Geometry: see drawing. Coordinates: mm, zero at the bounding-box minimum. A direction names the side the tool comes from. Coordinates: 2 decimals unless noted, no trailing zeros. Order: outer loops, then holes, each group sorted by start corner. A loop starts at its lowest first (then second) coordinate and runs counter-clockwise, first axis right, second up.
Item 1: Section D-D on y = 6. Return the cut outline in (x, z), then the cut area to 3 significant figures.
Item 2: Section A-A on x = 11.25. Return the cut outline in (y, z), then the cut area to 3 significant figures.
Item 3: Mould query, pull axis X, two halves, no side actions, for the marked faces 1, 2 and 3. Classes: released by +X, released by -X, zero draft, split by the parting line, or undercut.
Item 4: Reachability of the marked faces 4, 5, 6, 7 and 8 from +Z, -Z, +X, -X, +Y, -Y: full face, straight path, thin tool, end or side. Return the list, or none.
Item 5: Contact query for flat-ended pins moving along their axis: P1, Ø2, axis at y = 11, z = 9.5, coming from the -X side (3 decimals); P2, Ø1.2, axis at y = 9, z = 11, coming from the +X side (3 decimals); P3, Ø1.2, axis at x = 10.5, y = 9, coming from the +Z side; P4, Ø4, axis at x = 12, z = 2.5, coming from the -Y side. Output: stop coordinate, or through.
Item 6: Section C-C on z = 11. Return the cut outline in (x, y) (3 decimals), then the cut area to 3 significant figures.
Item 7: Section B-B on y = 10. Return the cut outline in (x, z) (3 decimals), then the cut area to 3 significant figures.
Item 8: Ray query, line 1 (Z direction, x = 6, y = 9.25); line 2 (X direction, y = 11, z = 10.75) (3 decimals); line 3 (Z direction, x = 12, y = 2). Return the intervals inside material, ascending.
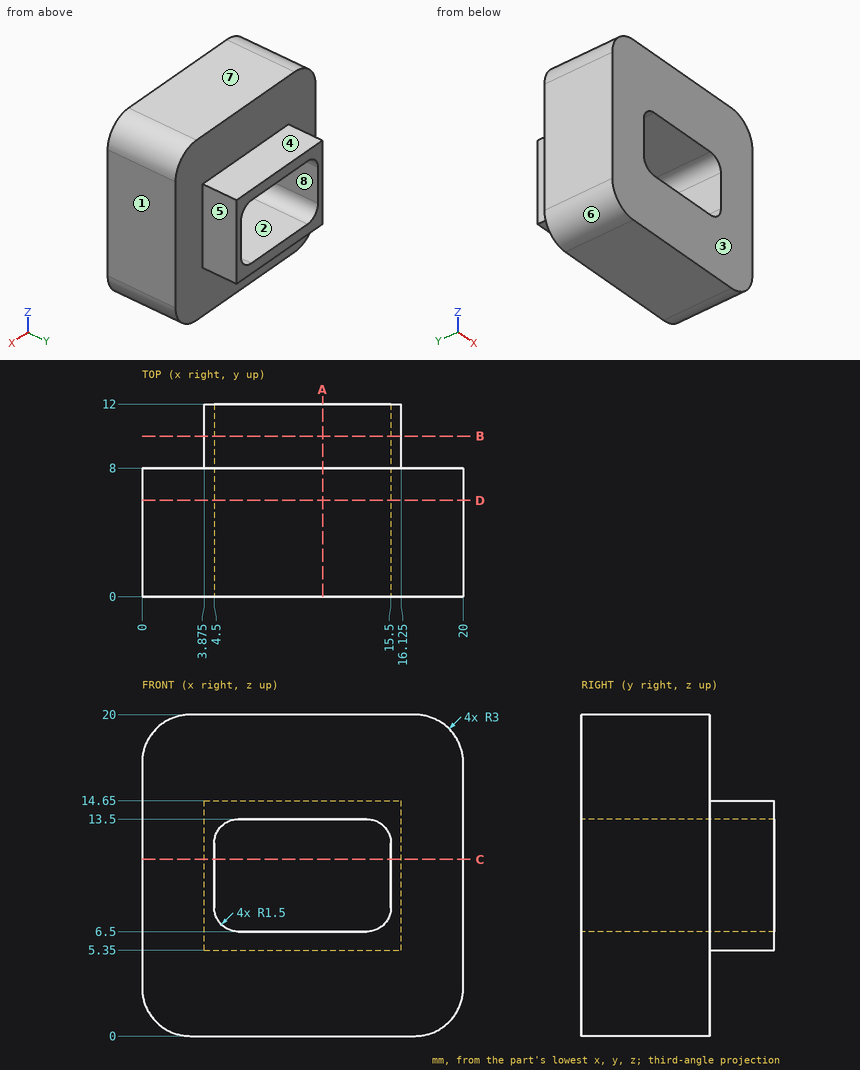
Answer list:
1. outline: (0, 3) arc R3 ccw to (3, 0) - (17, 0) arc R3 ccw to (20, 3) - (20, 17) arc R3 ccw to (17, 20) - (3, 20) arc R3 ccw to (0, 17) - close; hole (4.5, 8) arc R1.5 ccw to (6, 6.5) - (14, 6.5) arc R1.5 ccw to (15.5, 8) - (15.5, 12) arc R1.5 ccw to (14, 13.5) - (6, 13.5) arc R1.5 ccw to (4.5, 12) - close
1. area: 317 mm2
2. outline: (0, 0) - (8, 0) - (8, 5.35) - (12, 5.35) - (12, 6.5) - (0, 6.5) - close; (0, 13.5) - (12, 13.5) - (12, 14.65) - (8, 14.65) - (8, 20) - (0, 20) - close
2. area: 113 mm2
3. face 1: released by +X
3. face 2: undercut
3. face 3: zero draft
4. face 4: +Z, +X, -X, +Y
4. face 5: +Z, -Z, +X, +Y
4. face 6: -Z, -X, +Y, -Y
4. face 7: +Z, +X, -X, +Y, -Y
4. face 8: +Y, -Y
5. P1: stops at x = 3.875
5. P2: stops at x = 16.125
5. P3: stops at z = 14.65
5. P4: stops at y = 0
6. outline: (0, 0) - (4.5, 0) - (4.5, 12) - (3.875, 12) - (3.875, 8) - (0, 8) - close; (15.5, 0) - (20, 0) - (20, 8) - (16.125, 8) - (16.125, 12) - (15.5, 12) - close
6. area: 77.0 mm2
7. outline: (3.875, 5.35) - (16.125, 5.35) - (16.125, 14.65) - (3.875, 14.65) - close; hole (4.5, 8) arc R1.5 ccw to (6, 6.5) - (14, 6.5) arc R1.5 ccw to (15.5, 8) - (15.5, 12) arc R1.5 ccw to (14, 13.5) - (6, 13.5) arc R1.5 ccw to (4.5, 12) - close
7. area: 38.9 mm2
8. line 1: z = 5.35 to 6.5, 13.5 to 14.65
8. line 2: x = 3.875 to 4.5, 15.5 to 16.125
8. line 3: z = 0 to 6.5, 13.5 to 20
